Design review of the part built by this model. Coordinates are the model's own, in mm. A direction names the side the tool comes from. Give positions to 0.01 mm unless a question says otherwise; leave off trailing zeros. Order: outer loops, then holes, each group sorted by start corner. A loop starts at its lowest first (then second) coordinate and runs counter-clockwise, first axis right, second up. Notation, with made-up numbers: (-40, -6) -> (3, -6) arc R15 cw to (3, 2) -> close; hole circle Ø2 at (4.5, 14.25). An arc over 180 degrees is marked (long way). Answer in a Markdown table with one row per item. Add a question column.
```python
from build123d import *

# Parameters (mm, degrees)
SKETCH1_R               = 5.5
BOSS_EXTRUDE1_DEPTH     = 14
CUT_EXTRUDE3_DEPTH      = 6.5
CUT_EXTRUDE3_DEPTH_BACK = 6.5
CUT_EXTRUDE4_DEPTH      = 6.5000001
CUT_EXTRUDE4_DEPTH_BACK = 6.5000001
SKETCH5_R               = 3
CUT_EXTRUDE7_DEPTH      = 15.0000001
CUT_EXTRUDE7_DEPTH_BACK = 14
SKETCH6_R               = 1
CUT_EXTRUDE8_DEPTH      = 6.5000001
CUT_EXTRUDE8_DEPTH_BACK = 6.5000001


with BuildPart() as part:
    # Sketch1 → Boss-Extrude1 (new body)
    with BuildSketch(Plane(origin=(0, 0, 0), x_dir=(1, 0, 0), z_dir=(0, 1, 0))):
        Circle(SKETCH1_R)
    extrude(amount=BOSS_EXTRUDE1_DEPTH)

    # Sketch3 → Cut-Extrude3 (cut, two sides)
    with BuildSketch(Plane.XY) as cut_extrude3_sk:
        with BuildLine():
            Line((45.232137495, 10), (5.5, 10))
            ThreePointArc((5.5, 10), (4.209777241, 9.528177094), (3.528311133, 8.335325231))
            Line((3.528311133, 8.335325231), (2.464611084, 2.080843461))
            ThreePointArc((2.464611084, 2.080843461), (0, 0), (-2.464611084, 2.080843461))
            Line((-2.464611084, 2.080843461), (-3.528311133, 8.335325231))
            ThreePointArc((-3.528311133, 8.335325231), (-4.209777241, 9.528177094), (-5.5, 10))
            Line((-5.5, 10), (-45.232137495, 10))
            Line((-45.232137495, 10), (-45.232137495, -69.464274989))
            Line((-45.232137495, -69.464274989), (45.232137495, -69.464274989))
            Line((45.232137495, -69.464274989), (45.232137495, 10))
        make_face()
    extrude(amount=CUT_EXTRUDE3_DEPTH, mode=Mode.SUBTRACT)
    extrude(cut_extrude3_sk.sketch, amount=-CUT_EXTRUDE3_DEPTH_BACK, mode=Mode.SUBTRACT)

    # Sketch4 → Cut-Extrude4 (cut, two sides)
    with BuildSketch(Plane(origin=(0, 0, 0), x_dir=(0, 0, -1), z_dir=(1, 0, 0))) as cut_extrude4_sk:
        with BuildLine():
            Line((4.004785901, 0), (-3.995214099, 0))
            Line((-3.995214099, 0), (-2.98912449, 9.074785729))
            ThreePointArc((-2.98912449, 9.074785729), (-2.662225586, 9.709641809), (-1.995214099, 9.964594376))
            Line((-1.995214099, 9.964594376), (2.004785901, 9.964594376))
            ThreePointArc((2.004785901, 9.964594376), (2.671797388, 9.709641809), (2.998696292, 9.074785729))
            Line((2.998696292, 9.074785729), (4.004785901, 0))
        make_face()
    extrude(amount=CUT_EXTRUDE4_DEPTH, mode=Mode.SUBTRACT)
    extrude(cut_extrude4_sk.sketch, amount=-CUT_EXTRUDE4_DEPTH_BACK, mode=Mode.SUBTRACT)

    # Sketch5 → Cut-Extrude7 (cut, two sides)
    with BuildSketch(Plane(origin=(0, 0, 0), x_dir=(1, 0, 0), z_dir=(0, 1, 0))) as cut_extrude7_sk:
        Circle(SKETCH5_R)
    extrude(amount=CUT_EXTRUDE7_DEPTH, mode=Mode.SUBTRACT)
    extrude(cut_extrude7_sk.sketch, amount=-CUT_EXTRUDE7_DEPTH_BACK, mode=Mode.SUBTRACT)

    # Sketch6 → Cut-Extrude8 (cut, two sides)
    with BuildSketch(Plane.XY) as cut_extrude8_sk:
        with Locations((0, 3)):
            Circle(SKETCH6_R)
    extrude(amount=CUT_EXTRUDE8_DEPTH, mode=Mode.SUBTRACT)
    extrude(cut_extrude8_sk.sketch, amount=-CUT_EXTRUDE8_DEPTH_BACK, mode=Mode.SUBTRACT)


solid = part.part
```
1) Add section C-C, the plane y = 8. Write out the cut boundary in (x, z), and give its area (3 significant figures).
2) Add section B-B, the plane x = -2. Write out the cut boundary in (y, z), and give its area (3 significant figures).
3) Clearance check with flat-ended pins moving along their axes: P1, Ø3, axis at x = -3, z = 0, coming from the -Y side; P2, Ø4, axis at x = 2.5, y = 12.5, coming from the -Z side; P3, Ø2, axis at y = 4.5, z = -3, coming from the +X side; P4, Ø3, axis at x = -1.5, z = -0.5, coming from the +Y side. State where each tip first meets the part, or that it passes through.
4) Mouldability with a two-part tool opening along Y and no side actions: class faces 1 (the face through (0, 4, 5)), 2 (the face through (2.64, 9.72, -2.66)), 3 (the face through (2.4, 14, 2.4)), 4 (the face through (0, 4, -5)) as +Y half, -Y half, draft (parallel to the pull), parting line (faces both ways), or undercut.
5) For L1, parallel to Z at x = 0, y = 12.3; L2, parallel to Y at x = 0, z = 4.25, list the stretches that pass through material, from the lowest coordinate up.
6) Machinability: for faces 5 (the face through (-3.9, 9.2, 3.4)), 6 (the face through (-2.66, 9.7, 2.67)), which of the approach directions +Z, -Z, +X, -X, +Y, -Y give a long, thin tool a straight path to every point of the face, cutting with its end or side? Answer none if there is none.
7) Add section D-D, the plane y = 3. Write out the cut boundary in (x, z).
8) Add section A-A, the plane z = 0. Write out the cut boundary in (x, y).
Verdict:
| question | item | result |
|---|---|---|
| 1 | outline | (-3.47, -4.27) arc R5.5 ccw to (3.47, -4.27) -> (3.47, -3.12) -> (-3.47, -3.12) -> close; (-3.47, 3.11) -> (3.47, 3.11) -> (3.47, 4.27) arc R5.5 ccw to (-3.47, 4.27) -> close |
| 1 | area | 27.7 mm2 |
| 2 | outline | (1, -5.12) -> (14, -5.12) -> (14, -2.24) -> (9.94, -2.24) arc R1 cw to (9.07, -3) -> (1, -3.89) -> close; (1, 3.88) -> (9.07, 2.99) arc R1 cw to (9.94, 2.24) -> (14, 2.24) -> (14, 5.12) -> (1, 5.12) -> close |
| 2 | area | 54.7 mm2 |
| 3 | P1 | stops at y = 9.96 |
| 3 | P2 | stops at z = -5.48 |
| 3 | P3 | stops at x = 3.03 |
| 3 | P4 | stops at y = 14 |
| 4 | face 1 | undercut |
| 4 | face 2 | -Y half |
| 4 | face 3 | +Y half |
| 4 | face 4 | undercut |
| 5 | L1 | z = -5.5 to -3, 3 to 5.5 |
| 5 | L2 | y = 0 to 2, 4 to 14 |
| 6 | face 5 | +Z, -Z, -X, -Y |
| 6 | face 6 | +X, -X, -Y |
| 7 | outline | (-2.62, -4.84) arc R5.5 ccw to (-1, -5.41) -> (-1, -3.67) -> (-2.62, -3.67) -> close; (-2.62, 3.66) -> (-1, 3.66) -> (-1, 5.41) arc R5.5 ccw to (-2.62, 4.84) -> close; (1, -5.41) arc R5.5 ccw to (2.62, -4.84) -> (2.62, -3.67) -> (1, -3.67) -> close; (1, 3.66) -> (2.62, 3.66) -> (2.62, 4.84) arc R5.5 ccw to (1, 5.41) -> close |
| 8 | outline | (-5.5, 10) arc R2 cw to (-5.13, 9.96) -> (-3, 9.96) -> (-3, 14) -> (-5.5, 14) -> close; (3, 9.96) -> (5.13, 9.96) arc R2 cw to (5.5, 10) -> (5.5, 14) -> (3, 14) -> close |
